Could you check a few things on this drawing? It's one solid part, dimensions in mm from its lowest x, y, z. A direction names the side the tool comes from. Round coordinates to 2 decimals unless told otherwise and drop trailing zeros. Order: outer loops, then holes, each group sorted by start corner. A loop starts at its lowest first (then second) coordinate and runs counter-clockwise, first axis right, second up. Notation, with made-up numbers: (24.25, 57.5) - (79.25, 57.5) arc R25 ccw to (79.25, 84.5) - close; hole circle Ø6 at (53.5, 23.25). An arc over 180 degrees is marked (long way). Use one line per item in the form item = value.
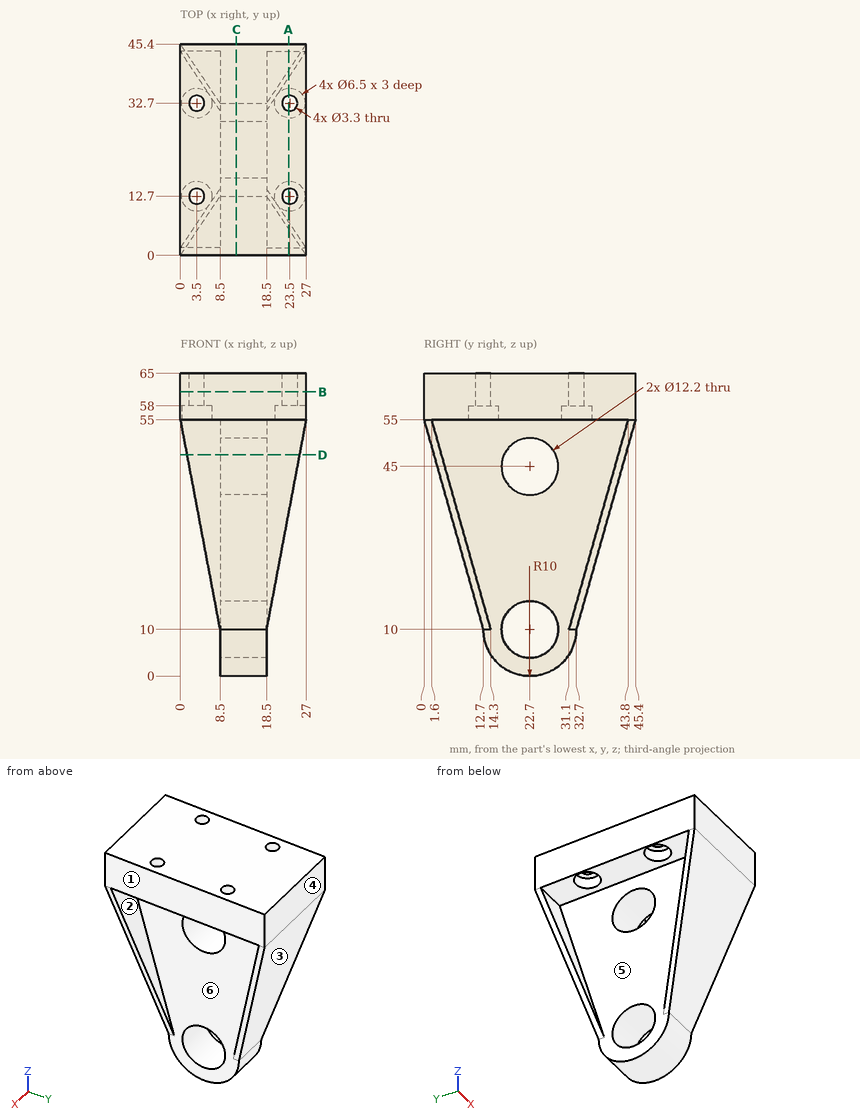
Item 1: Will these pins go through, and if not, where does the flat tip stop? P1, Ø2.5, axis at x = 3.5, y = 32.7, coming from the -Z side; P2, Ø1.5, axis at y = 38.5, z = 49, coming from the +X side; P3, Ø4, axis at x = 4.5, y = 14.5, coming from the -Z side; P4, Ø12.5, axis at y = 27.5, z = 39, coming from the -X side.
Found:
P1 = through
P2 = 18.5
P3 = 55
P4 = 8.5
Item 2: Imagine slicing it at C-C on x = 12. Please give me the cut outline in (y, z).
Found:
outline = (0, 55) - (12.7, 10) arc R10 ccw to (32.7, 10) - (45.4, 55) - (45.4, 65) - (0, 65) - close; hole circle Ø12.2 at (22.7, 10); hole circle Ø12.2 at (22.7, 45)
Item 3: For the marked faces 4, 5 and 6, which set-ups out of +Z, -Z, +X, -X, +Y, -Y let a thin tool reach every point of the face, with its end or its side?
Found:
face_4 = +Z, -Z, +X, -X, +Y
face_5 = -X
face_6 = +X
Item 4: Imagine slicing it at A-A on x = 23.25. Please give me the cut outline in (y, z).
Found:
outline = (0, 55) - (5.6, 35.15) - (7.2, 35.15) - (1.6, 55) - (9.46, 55) - (9.46, 58) - (11.07, 58) - (11.07, 65) - (0, 65) - close; (14.33, 58) - (15.94, 58) - (15.94, 55) - (29.46, 55) - (29.46, 58) - (31.07, 58) - (31.07, 65) - (14.33, 65) - close; (34.33, 58) - (35.94, 58) - (35.94, 55) - (43.8, 55) - (38.2, 35.15) - (39.8, 35.15) - (45.4, 55) - (45.4, 65) - (34.33, 65) - close
Item 5: I need wall thicknesses on L1, parallel to X at y = 12.7, z = 61.25; L2, parallel to Y at x = 3.5, z = 60.75; L3, parallel to Z at x = 16.75, y = 25. Which ranges of each line are inside material? Lowest first, please.
Found:
L1 = 0 to 1.85, 5.15 to 21.85, 25.15 to 27
L2 = 0 to 11.05, 14.35 to 31.05, 34.35 to 45.4
L3 = 0.27 to 4.35, 15.65 to 39.35, 50.65 to 65
Item 6: Imagine slicing it at D-D on z = 47.5. Please give me the cut outline in (x, y), plus the area to 3 significant figures.
Found:
outline = (1.42, 2.12) - (25.58, 2.12) - (25.58, 3.72) - (18.5, 3.72) - (18.5, 17.14) - (8.5, 17.14) - (8.5, 3.72) - (1.42, 3.72) - close; (1.42, 41.68) - (8.5, 41.68) - (8.5, 28.26) - (18.5, 28.26) - (18.5, 41.68) - (25.58, 41.68) - (25.58, 43.28) - (1.42, 43.28) - close
area = 346 mm2
Item 7: Imagine slicing it at B-B on z = 61. Please give me the cut outline in (x, y), plus the area to 3 significant figures.
Found:
outline = (0, 0) - (27, 0) - (27, 45.4) - (0, 45.4) - close; hole circle Ø3.3 at (3.5, 12.7); hole circle Ø3.3 at (3.5, 32.7); hole circle Ø3.3 at (23.5, 12.7); hole circle Ø3.3 at (23.5, 32.7)
area = 1,190 mm2
Item 8: If we mould it in two halves opening along Z, with no side actions, what happens to the marked faces 1, 2 and 3? For each: released by +Z, released by -Z, zero draft, split by the parting line, or undercut.
Found:
face_1 = zero draft
face_2 = undercut
face_3 = released by -Z
